Read the model definition and answer for the solid it produces. Units are mm, in the model's axes. A direction names the side the tool comes from. Coordinates: 2 decimals unless noted, no trailing zeros. Order: outer loops, then holes, each group sorted by start corner. A loop starts at its lowest first (then second) coordinate and runs counter-clockwise, first axis right, second up. Notation, with made-up numbers: (56, 45.25) - (65, 45.25) arc R26 cw to (65, 75.25) - close; hole circle Ø9 at (-6.5, 31). An arc over 180 degrees is marked (long way). Answer as a JSON object with one key per item and string values. Group by question number.
from build123d import *

# Parameters (mm, degrees)
CYLINDER001_R         = 2
CYLINDER001_DEPTH     = 10
CYLINDER002_R         = 2
CYLINDER002_DEPTH     = 10
TORUS_R               = 2
TORUS_ANGLE           = 120
TORUS_PLACEMENT_ANGLE = 255
CYLINDER_R            = 15
CYLINDER_DEPTH        = 3


with BuildPart() as cilindro001:
    # Cylinder001 → Cylinder001 (new body)
    with BuildSketch(Plane(origin=(0, 8, 1), x_dir=(1, 0, 0), z_dir=(0, 0, 1))):
        Circle(CYLINDER001_R)
    extrude(amount=CYLINDER001_DEPTH)


with BuildPart() as fusion:
    # Cylinder002 → Cylinder002 (new body)
    with BuildSketch(Plane(origin=(-8, 0, 1), x_dir=(1, 0, 0), z_dir=(0, 0, 1))):
        Circle(CYLINDER002_R)
    extrude(amount=CYLINDER002_DEPTH)

    # Fusion: union Cilindro001
    add(cilindro001.part)


with BuildPart() as toro:
    # Torus → Torus (revolve)
    with BuildSketch(Plane.XZ):
        with Locations((10, 0)):
            Circle(TORUS_R)
    revolve(axis=Axis((0, 0, 0), (0, 0, 1)), revolution_arc=TORUS_ANGLE)


with BuildPart() as toro_1:
    # Torus placement: moved
    add(toro.part.moved(Location((0, 0, 3))).rotate(Axis((0, 0, 3), (0, 0, 1)), TORUS_PLACEMENT_ANGLE))


with BuildPart() as cut001:
    # Cylinder → Cylinder (new body)
    with BuildSketch(Plane.XY):
        Circle(CYLINDER_R)
    extrude(amount=CYLINDER_DEPTH)

    # Cut: cut Toro
    add(toro_1.part, mode=Mode.SUBTRACT)

    # Cut001: cut Fusion
    add(fusion.part, mode=Mode.SUBTRACT)


solid = cut001.part
1. For a pull along X with two mould halves and no side action, classify faces 1 (the cylindrical face through (0, 10, 2)), 2 (the cylindrical face through (-14.985, 0.66, 1.479)), 3 (the flat face through (0, 0, 3)), 4 (the cylindrical face through (-9.6, -1.2, 2)) as pulls with the +X half, pulls with the -X half, needs draft (parallel to the pull), parting line crosses it, or undercut.
2. A cutting plane is placed at C-C on z = 2.4. Write down the section's boundary in (x, y), and give its area (3 significant figures).
3. A cutting plane is placed at A-A on y = 0. Write down the section's boundary in (x, z), and give its area (3 significant figures).
4. A cutting plane is placed at B-B on x = 0. Write down the section's boundary in (y, z), and give its area (3 significant figures).
5. Straight lines are drawn through the part: L1, parallel to Y at x = 0, z = 2.2; L2, parallel to Z at x = -9.75, y = -0.25; L3, parallel to Y at x = -8.5, z = 1.15. For each, find the intervals that lie inside material, in ascending order.
6. Given pin 1 (1.2 mm diameter, centred on x = -0.5, y = 7, fed in from +Z); pin 2 (1 mm diameter, centred on x = 2.5, z = 1, fed in from +Y), each flat-ended and moving along its own axis, determine where each tip first touches the part or whether it passes through.
7. For faces 5 (the flat face through (0, 0, 0)), 6 (the flat face through (-2.58, -9.63, 2.24)), determine the directions among +Z, -Z, +X, -X, +Y, -Y from which every point of the face is accessible in a straight line to the end or side of a thin tool.
8. A cutting plane is placed at D-D on z = 0.35. Write down the section's boundary in (x, y).
Derived:
{
 "1": {"face 1": "undercut", "face 2": "parting line crosses it", "face 3": "needs draft", "face 4": "undercut"},
 "2": {"outline": "circle Ø30 at (0, 0); hole circle Ø4 at (-8, 0); hole (-3.08, -11.5) arc R11.91 ccw to (11.5, 3.08) - (7.82, 2.09) arc R8.09 cw to (-2.09, -7.82) - close; hole circle Ø4 at (0, 8)", "area": "602 mm2"},
 "3": {"outline": "(-15, 0) - (15, 0) - (15, 3) - (12, 3) arc R2 cw to (8, 3) - (-6, 3) - (-6, 1) - (-10, 1) - (-10, 3) - (-15, 3) - close", "area": "75.7 mm2"},
 "4": {"outline": "(-15, 0) - (15, 0) - (15, 3) - (10, 3) - (10, 1) - (6, 1) - (6, 3) - (-8, 3) arc R2 cw to (-12, 3) - (-15, 3) - close", "area": "75.7 mm2"},
 "5": {"L1": "y = -15 to -11.83, -8.17 to 6, 10 to 15", "L2": "z = 0 to 1", "L3": "y = -12.36 to -1.94, 1.94 to 12.36"},
 "6": {"pin 1": "stops at z = 1", "pin 2": "stops at y = 14.87"},
 "7": {"face 5": "-Z, +X, -X, +Y, -Y", "face 6": "+Z"},
 "8": {"outline": "circle Ø30 at (0, 0)"}
}
